```python
from build123d import *

# Parameters (mm, degrees)
SKETCH2_R               = 2.5
SKETCH2_R_2             = 1.25
BOSS_EXTRUDE1_DEPTH     = 6.25
BOSS_EXTRUDE1_2_DEPTH   = 6.25
SKETCH3_R               = 2.5
SKETCH3_R_2             = 1.25
CUT_EXTRUDE1_DEPTH      = 5.05
BOSS_EXTRUDE2_DEPTH     = 6.25
CUT_EXTRUDE2_DEPTH      = 12.34392559
CUT_EXTRUDE2_DEPTH_BACK = 12.34392559
SKETCH6_R               = 1.25
BOSS_EXTRUDE3_DEPTH     = 11.001
SKETCH7_R               = 2.5
SKETCH7_R_2             = 1.25
CUT_EXTRUDE3_DEPTH      = 2.5
SCALE1_SCALE            = 1.5


with BuildPart() as part:
    # Sketch2 → Boss-Extrude1 (new, symmetric)
    with BuildSketch(Plane(origin=(0, 0, 0), x_dir=(0, 0, -1), z_dir=(1, 0, 0))):
        with Locations((6.630835, 0)):
            Circle(SKETCH2_R)
        with Locations((6.630835, 0)):
            Circle(SKETCH2_R_2, mode=Mode.SUBTRACT)
    extrude(amount=BOSS_EXTRUDE1_DEPTH, both=True)


with BuildPart() as body_2:
    # Sketch2 → Boss-Extrude1 2 (new, symmetric)
    with BuildSketch(Plane(origin=(0, 0, 0), x_dir=(0, 0, -1), z_dir=(1, 0, 0))):
        with Locations((-6.630835, 0)):
            Circle(SKETCH2_R)
        with Locations((-6.630835, 0)):
            Circle(SKETCH2_R_2, mode=Mode.SUBTRACT)
    extrude(amount=BOSS_EXTRUDE1_2_DEPTH, both=True)


with BuildPart() as cut_extrude1_tool:
    # Sketch3 → Cut-Extrude1 (new, symmetric)
    # profile 1 of 2: a face of its own
    with BuildSketch(Plane(origin=(0, 0, 0), x_dir=(0, 0, -1), z_dir=(1, 0, 0))):
        with Locations((6.630835, 0)):
            Circle(SKETCH3_R)
        with Locations((6.630835, 0)):
            Circle(SKETCH3_R_2, mode=Mode.SUBTRACT)
    # profile 2 of 2: a face of its own
    with BuildSketch(Plane(origin=(0, 0, 0), x_dir=(0, 0, -1), z_dir=(1, 0, 0))):
        with Locations((-6.630835, 0)):
            Circle(SKETCH3_R)
        with Locations((-6.630835, 0)):
            Circle(SKETCH3_R_2, mode=Mode.SUBTRACT)
    extrude(amount=CUT_EXTRUDE1_DEPTH, both=True)


with BuildPart() as part_1:
    add(part.part)

    # Cut-Extrude1: cut by cut_extrude1_tool
    add(cut_extrude1_tool.part, mode=Mode.SUBTRACT)


with BuildPart() as body_2_1:
    add(body_2.part)

    # Cut-Extrude1: cut by cut_extrude1_tool
    add(cut_extrude1_tool.part, mode=Mode.SUBTRACT)


with BuildPart() as cut_extrude1_piece_1:
    # of the separate pieces the step leaves, piece 1, a body of its own (cut_extrude1_pieces)
    add(part_1.part.solids().sort_by_distance((-6.25, 0, -9.130835))[0])



with BuildPart() as cut_extrude1_piece_2:
    # of the separate pieces the step leaves, piece 2, a body of its own (cut_extrude1_pieces)
    add(part_1.part.solids().sort_by_distance((5.05, 0, -9.130835))[0])


with BuildPart() as cut_extrude1_piece_1_of_body_2:
    # of the separate pieces the step leaves, piece 1, a body of its own (cut_extrude1_pieces_of_body_2)
    add(body_2_1.part.solids().sort_by_distance((-6.25, 0, 4.130835))[0])


with BuildPart() as cut_extrude1_piece_2_of_body_2:
    # of the separate pieces the step leaves, piece 2, a body of its own (cut_extrude1_pieces_of_body_2)
    add(body_2_1.part.solids().sort_by_distance((5.05, 0, 4.130835))[0])


with BuildPart() as cut_extrude1_piece_1_1:
    add(cut_extrude1_piece_1.part)

    add(cut_extrude1_piece_2.part)  # Boss-Extrude2 merges Cut-Extrude1 piece 2

    add(cut_extrude1_piece_1_of_body_2.part)  # Boss-Extrude2 merges Cut-Extrude1 piece 1 of body 2

    add(cut_extrude1_piece_2_of_body_2.part)  # Boss-Extrude2 merges Cut-Extrude1 piece 2 of body 2
    # Sketch4 → Boss-Extrude2 (add, symmetric)
    with BuildSketch(Plane(origin=(0, 0, 0), x_dir=(0, 0, -1), z_dir=(1, 0, 0))):
        with BuildLine():
            ThreePointArc((4.853650324, 1.758298788), (4.130835, 0), (4.853650324, -1.758298788))
            ThreePointArc((4.853650324, -1.758298788), (0, -0.947912117), (-4.853650324, -1.758298788))
            ThreePointArc((-4.853650324, -1.758298788), (-4.130835, 0), (-4.853650324, 1.758298788))
            ThreePointArc((-4.853650324, 1.758298788), (0, 0.947912117), (4.853650324, 1.758298788))
        make_face()
    extrude(amount=BOSS_EXTRUDE2_DEPTH, both=True)

    # Sketch5 → Cut-Extrude2 (cut, two sides: drawn at the far end of the back side and taken through both)
    with BuildSketch(Plane(origin=(0, 0, 0), x_dir=(1, 0, 0), z_dir=(0, 1, 0)).offset(-CUT_EXTRUDE2_DEPTH_BACK)):
        with BuildLine():
            Line((-5.05, 4.853650324), (5.05, 4.853650324))
            ThreePointArc((5.05, 4.853650324), (0, 0.25), (-5.05, 4.853650324))
        make_face()
        with BuildLine():
            Line((5.05, -4.853650324), (-5.05, -4.853650324))
            ThreePointArc((-5.05, -4.853650324), (0, -0.25), (5.05, -4.853650324))
        make_face()
    extrude(amount=CUT_EXTRUDE2_DEPTH + CUT_EXTRUDE2_DEPTH_BACK, mode=Mode.SUBTRACT)

    # Sketch6 → Boss-Extrude3 (add)
    with BuildSketch(Plane(origin=(-5.05, 0, 0), x_dir=(0, 0, -1), z_dir=(1, 0, 0))):
        with BuildLine():
            ThreePointArc((-4.853650324, 1.758298788), (-9.130835, 0), (-4.853650324, -1.758298788))
            ThreePointArc((-4.853650324, -1.758298788), (-4.130835, 0), (-4.853650324, 1.758298788))
        make_face()
        with Locations((-6.630835, 0)):
            Circle(SKETCH6_R, mode=Mode.SUBTRACT)
    extrude(amount=BOSS_EXTRUDE3_DEPTH)

    # Sketch7 → Cut-Extrude3 (cut, symmetric)
    with BuildSketch(Plane(origin=(0, 0, 0), x_dir=(0, 0, -1), z_dir=(1, 0, 0))):
        with Locations(Location((-6.630835, 0, 0), (0, 0, 44.693939637))):
            Circle(SKETCH7_R)
        with Locations((-6.630835, 0)):
            Circle(SKETCH7_R_2, mode=Mode.SUBTRACT)
    extrude(amount=CUT_EXTRUDE3_DEPTH, both=True, mode=Mode.SUBTRACT)


with BuildPart() as cut_extrude1_piece_1_2:
    # Scale1: scaled about (-1.5e-08, -4.9e-08, 2.005345841)
    add(cut_extrude1_piece_1_1.part.scale(SCALE1_SCALE).moved(Location((7e-09, 2.5e-08, -1.002672921))))


solid = cut_extrude1_piece_1_2.part
```
Verification items for the finished model (mm, model axes). A direction names the side the tool comes from. Coordinates: 2 decimals unless noted, no trailing zeros. Write each loop counter-clockwise with the first axis right and the second up, starting at its lowest first coordinate (ties: lowest second). Pieces come first, ordered by that corner, then holes. Notation, with made-up numbers: M 1.5,65.5 L 54.5,65.5 A21 ccw 54.5,82.5 Z; hole C 6,6 d7. An arc over 180 degrees is marked long. One line per item, written item: value.
Item 1: Mould release check, pull along Z, two halves, no side actions. Record for faces 1 (the cylindrical face through (0.16, -0.04, -1.38)), 2 (the flat face through (-3.75, -2, 10)), 3 (the cylindrical face through (8.488, -0.124, -14.697)): pulls with the +Z half, pulls with the -Z half, needs draft (parallel to the pull), parting line crosses it, or undercut.
Check sheet entries:
face 1: pulls with the -Z half
face 2: needs draft
face 3: undercut
Item 2: Scan lines: line 1 along X through (y, z) = (-0.5, 5.5) (3 decimals); line 2 along Z through (x, y) = (-4.75, 1); line 3 along Z through (x, y) = (8.25, 1) (1 decimal). Record each from-to range of solid material in increasing order.
Check sheet entries:
line 1: x = -9.375 to -3.75, 3.75 to 9.375
line 2: z = -3.04 to 1.04, 5.33 to 7.36, 10.53 to 12.56
line 3: z = -14.6 to -12.5, -9.4 to 7.4, 10.5 to 12.6
Item 3: Section check A-A, the plane y = 0. State how many separate pieces and enclosed holes the cut face has, plus the area to 3 significant figures.
Check sheet entries:
separate pieces: 5
enclosed holes: 0
area: 160 mm^2
Item 4: Section check C-C, the plane z = -6.5. Record the boundary of the cut face in (x, y) (3 decimals), plus the area to 3 significant figures.
Check sheet entries:
outline: M -9.375,-2.107 L -7.19,-2.107 L -7.19,2.107 L -9.375,2.107 Z; M 7.19,-2.107 L 9.375,-2.107 L 9.375,2.107 L 7.19,2.107 Z
area: 18.4 mm^2
Item 5: Section check D-D, the plane y = 3. Record the boundary of the cut face in (x, z) (3 decimals), plus the area to 3 significant figures.
Check sheet entries:
outline: M -9.375,-13.199 L -7.575,-13.199 L -7.575,-8.699 L -9.375,-8.699 Z; M -9.375,6.694 L -3.75,6.694 L -3.75,11.194 L -9.375,11.194 Z; M 3.75,6.694 L 9.375,6.694 L 9.375,11.194 L 3.75,11.194 Z; M 7.575,-13.199 L 9.375,-13.199 L 9.375,-8.699 L 7.575,-8.699 Z
area: 66.8 mm^2
Item 6: Section check B-B, the plane x = 5. Record the boundary of the cut face in (y, z) (3 decimals).
Check sheet entries:
outline: C 0,8.944 d7.5; M -1.535,-3.252 L 1.535,-3.252 A22.41 cw 1.535,1.246 L -1.535,1.246 A22.41 cw Z; hole C 0,8.944 d3.75
Item 7: Gauge pin test, flat ends, axial feed: pin 1 Ø4.5 at (y, z) = (0, 8.94) entering from +X (3 decimals); pin 2 Ø3 at (y, z) = (0, -10.95) entering from +X; pin 3 Ø5 at (x, z) = (-7.5, -2.5) entering from +Y; pin 4 Ø3 at (x, z) = (5.5, -4.5) entering from -Y. Record the tip position at first contact, or that the pin passes through.
Check sheet entries:
pin 1: stops at x = 9.375
pin 2: passes through
pin 3: stops at y = 1.78
pin 4: stops at y = -1.86
Item 8: Access from +Z, -Z, +X, -X, +Y, -Y to the whole of each face (thin tool, end or side, straight path). Record for faces 4 (the cylindrical face through (-8.462, -0.124, -14.697)), 5 (the flat face through (3.75, -2, 10)).
Check sheet entries:
face 4: +X, -X
face 5: +Z, +Y, -Y
